Model file for the job. Use its own axes, mm. A direction names the side the tool comes from. Give positions to 0.01 mm unless a question says otherwise; leave off trailing zeros. Write each loop counter-clockwise with the first axis right and the second up, starting at its lowest first coordinate (ties: lowest second). Pieces come first, ordered by that corner, then holes. Notation, with made-up numbers: (18.5, -28) - (59.5, -28) arc R19 cw to (59.5, -10) - close; hole circle Ø2 at (66.25, 82.5). An arc over 180 degrees is marked (long way). One line per item, written item: value. Start each with the question number.
(1) Drop a flat-ended pin along its axis: P1, Ø2.5, axis at x = -26, y = 2, coming from the +Z side. Give the stop position or say it passes through.
(2) Probe L1, parallel to Z at x = 83, y = 1.1; L2, parallel to X at y = 3, z = 3.5; L3, parallel to X at y = 2.8, z = 9.5. List the from-to ranges inside material, lowest first.
(3) 3-axis set-ups, long thin cutter, end or side, ignore diameter. For faces 4 (the face through (-2, 3, -19.05)), 5 (the face through (117.5, 2.6, -3.6)): which of +Z, -Z, +X, -X, +Y, -Y reach the whole face in a straight line?
(4) Mould opens along X. For faces 1 (the face through (-133.35, 3, 7)), 2 (the face through (-1, 5.08, -13)), 3 (the face through (-117.5, 2.6, -3.6)) say: pulls with the +X half, pulls with the -X half, needs draft (parallel to the pull), parting line crosses it, or undercut.
(5) Cut at A-A, the plane z = 3. List the corners of the cut face in (x, y), and give its area (3 significant figures).
(6) Cut at B-B, the plane y = 0.8. List the corners of the cut face in (x, z), and give its area (3 significant figures).
(7) Cut at C-C, the plane z = -8.5. List the corners of the cut face in (x, y).
(8) Cut at D-D, the plane x = 6.5. List the corners of the cut face in (y, z).
from build123d import *

# Parameters (mm, degrees)
SKETCH1_W          = 266.7
SKETCH1_H          = 38.1
BUMPER_BASE_DEPTH  = 5.08
CUT_EXTRUDE1_DEPTH = 135.79959718
FILLET1_R          = 13.97


with BuildPart() as part:
    # Sketch1 → Bumper-Base (new body)
    with BuildSketch(Plane(origin=(0, 0, 0), x_dir=(1, 0, 0), z_dir=(0, 1, 0))):
        Rectangle(SKETCH1_W, SKETCH1_H)
    extrude(amount=BUMPER_BASE_DEPTH)

    # Sketch2 → Cut-Extrude1 (cut, symmetric)
    with BuildSketch(Plane(origin=(0, 5.08, 0), x_dir=(1, 0, 0), z_dir=(0, 1, 0))):
        with BuildLine():
            Line((0, 12.7), (-95.25, 12.7))
            ThreePointArc((-95.25, 12.7), (-117.700640303, 3.400640303), (-127, -19.05))
            Line((-127, -19.05), (-95.25, -19.05))
            Line((-95.25, -19.05), (0, -19.05))
            Line((0, -19.05), (0, 12.7))
        make_face()
    cut_extrude1 = extrude(amount=CUT_EXTRUDE1_DEPTH, both=True, mode=Mode.SUBTRACT)

    # Mirror1: Cut-Extrude1 across plane
    add(cut_extrude1.mirror(Plane(origin=(0, 0, 0), x_dir=(0, 0, 1), z_dir=(1, 0, 0))), mode=Mode.SUBTRACT)

    # Fillet1
    fillet1_edges = [part.edges().sort_by_distance(p)[0] for p in [
        (-133.35, 2.54, -19.05),
        (133.35, 2.54, -19.05),
    ]]
    fillet(fillet1_edges, radius=FILLET1_R)


solid = part.part
Answers follow:
1. P1: stops at z = -12.7
2. L1: z = -19.05 to -12.7
2. L2: x = -133.35 to -122.93, 122.93 to 133.35
2. L3: x = -133.35 to -125.53, 125.53 to 133.35
3. face 4: -Z, +X, -X, +Y, -Y
3. face 5: +Z, +Y, -Y
4. face 1: pulls with the -X half
4. face 2: needs draft
4. face 3: undercut
5. outline: (-133.35, 0) - (-122.64, 0) - (-122.64, 5.08) - (-133.35, 5.08) - close; (122.64, 0) - (133.35, 0) - (133.35, 5.08) - (122.64, 5.08) - close
5. area: 109 mm²
6. outline: (-133.35, -5.08) arc R13.97 ccw to (-119.38, -19.05) - (119.38, -19.05) arc R13.97 ccw to (133.35, -5.08) - (133.35, 19.05) - (127, 19.05) arc R31.75 cw to (95.25, -12.7) - (-95.25, -12.7) arc R31.75 cw to (-127, 19.05) - (-133.35, 19.05) - close
6. area: 2,450 mm²
7. outline: (-132.92, 0) - (-111.03, 0) - (-111.03, 5.08) - (-132.92, 5.08) - close; (111.03, 0) - (132.92, 0) - (132.92, 5.08) - (111.03, 5.08) - close
8. outline: (0, -19.05) - (5.08, -19.05) - (5.08, -12.7) - (0, -12.7) - close
